Source: CAD feature listing. Evaluate the final solid. Frame: model axes, mm. A direction names the side the tool comes from. Coordinates: 2 decimals unless noted, no trailing zeros. Loops run counter-clockwise (first coordinate to the right, second up) from the corner with the lowest first, then second, coordinate; pieces in that order, holes last. Notation, with made-up numbers: (38.5, -28) -> (51.5, -28) arc R16 cw to (51.5, 0) -> close; hole circle Ø10 at (22, 37). An arc over 180 degrees is marked (long way). Answer as CSV lines item,"result".
from build123d import *

# Parameters (mm, degrees)
BOSS_EXTRUDE1_START = 10.16
SKETCH3_R           = 3.175
BOSS_EXTRUDE1_DEPTH = 5.08
SKETCH4_R           = 0.635
CUT_EXTRUDE1_DEPTH  = 10.588339362


with BuildPart() as part:
    # Sketch1 → Revolve1 (revolve)
    with BuildSketch(Plane(origin=(0, 0, 0), x_dir=(0, 0, -1), z_dir=(1, 0, 0))):
        with BuildLine():
            Line((-76.2, 2.8321), (76.2, 2.8321))
            Line((76.2, 2.8321), (81.001685274, 3.678766667))
            Line((81.001685274, 3.678766667), (81.001685274, 5.3721))
            Line((81.001685274, 5.3721), (80.493685274, 5.385402448))
            Line((80.493685274, 5.385402448), (80.493685274, 5.893402448))
            Line((80.493685274, 5.893402448), (74.143685274, 5.893402448))
            Line((74.143685274, 5.893402448), (74.143685274, 5.55168305))
            Line((74.143685274, 5.55168305), (-60.96, 9.089497556))
            Line((-60.96, 9.089497556), (-60.96, 9.588339362))
            Line((-60.96, 9.588339362), (-80.01, 9.588339362))
            Line((-80.01, 9.588339362), (-84.333416613, 2.099962126))
            ThreePointArc((-84.333416613, 2.099962126), (-85.257877242, 1.477131543), (-86.317456021, 1.823308084))
            ThreePointArc((-86.317456021, 1.823308084), (-89.075761951, 2.339152699), (-90.625830312, 0))
            Line((-90.625830312, 0), (-85.545830312, 0))
            Line((-85.545830312, 0), (-76.2, 0))
            Line((-76.2, 0), (-76.2, 2.8321))
        make_face()
    revolve(axis=Axis((0, 0, 101.6), (0, 0, -1)))

    # Sketch3 → Boss-Extrude1 (add, symmetric)
    with BuildSketch(Plane(origin=(0, 0, 0), x_dir=(0, 0, -1), z_dir=(1, 0, 0)).offset(BOSS_EXTRUDE1_START)):
        Circle(SKETCH3_R)
    boss_extrude1 = extrude(amount=BOSS_EXTRUDE1_DEPTH, both=True)

    # Mirror1: Boss-Extrude1 across plane
    add(boss_extrude1.mirror(Plane(origin=(0, 0, 0), x_dir=(0, 0, 1), z_dir=(1, 0, 0))))

    # Sketch4 → Cut-Extrude1 (cut, through all)
    with BuildSketch(Plane(origin=(0, 0, 0), x_dir=(1, 0, 0), z_dir=(0, 1, 0))):
        with Locations((0, -67.31)):
            Circle(SKETCH4_R)
    extrude(amount=CUT_EXTRUDE1_DEPTH, mode=Mode.SUBTRACT)


solid = part.part
(1) Cut plane B-B (x = -12). Return the cut outline in (y, z) (3 decimals), then the cut area to 3 significant figures.
Computed values:
outline,"circle Ø6.35 at (0, 0)"
area,"31.7 mm^2"
(2) Material intervals for L1, parallel to X at y = 0, z = -42.5; L2, parallel to X at y = 6, z = 67.31 (3 decimals); L3, parallel to X at y = 6.75, z = 68.5, sorted ascending. Write a range as [from, to].
Computed values:
L1,"[-6.38, -2.83], [2.83, 6.38]"
L2,"[-7.479, -0.635], [0.635, 7.479]"
L3,"[-6.81, 6.81]"
(3) Cut plane A-A (z = 0). Return the cut outline in (x, y) (3 decimals).
Computed values:
outline,"(-15.24, -3.175) -> (-6.787, -3.175) arc R7.493 ccw to (6.787, -3.175) -> (15.24, -3.175) -> (15.24, 3.175) -> (6.787, 3.175) arc R7.493 ccw to (-6.787, 3.175) -> (-15.24, 3.175) -> close; hole circle Ø5.664 at (0, 0)"
(4) Draft query along Y for faces 1 (the cylindrical face through (-1.72, -2.25, -1.07)), 2 (the cylindrical face through (8.085, 5.155, 70.618)), 3 (the flat face through (15.24, 0, 0)). Return one class per face: released by +Y, released by -Y, zero draft, split by the parting line, or undercut.
Computed values:
face 1,"undercut"
face 2,"split by the parting line"
face 3,"zero draft"
(5) Cut plane D-D (z = 62.5). Return the cut outline in (x, y).
Computed values:
outline,"circle Ø19.18 at (0, 0); hole circle Ø5.66 at (0, 0)"
(6) Pin query (flat end, axial travel): pin 1 Ø3.5 at (x, y) = (0, 0) entering from -Z; pin 2 Ø2 at (y, z) = (3, -54) entering from -X; pin 3 Ø2 at (x, z) = (0, 67.31) entering from +Y; pin 4 Ø5 at (x, z) = (4, 68.5) entering from -Y. Return the tip coordinate at first contact, or that it passes through.
Computed values:
pin 1,"z = 76.2"
pin 2,"x = -5.74"
pin 3,"y = 9.59"
pin 4,"y = -9.47"
(7) Access query for faces 4 (the cylindrical face through (-11.07, 0.14, 3.17)), 5 (the flat face through (0, 0, 76.2)), 6 (the conical face through (2.206, 7.006, -5.646)), 7 (the cylindrical face through (11.07, 0.14, 3.17)). Directions: +Z, -Z, +X, -X, +Y, -Y. A direction counts if a zero-diameter tool reaches every point of the face in a straight line with its end or side. Return the directions, or none.
Computed values:
face 4,"-X"
face 5,"-Z"
face 6,"none"
face 7,"+X"
